The listing builds one solid part. Answer for the finished solid, in the listing's coordinates (mm). Face numbers are marked on the shaded views. Coordinates: 2 decimals unless noted, no trailing zeros. Loops run counter-clockwise (first coordinate to the right, second up) from the corner with the lowest first, then second, coordinate; pieces in that order, holes last. Notation, with made-up numbers: (81, 28.25) - (101, 28.25) arc R24 ccw to (101, 52.25) - close; hole circle Ø5 at (47.25, -9). An arc over 180 degrees is marked (long way). Return JSON: item names as keys, results as strings. Group by question number.
1. Each of these flat-tipped pins is pushed along its axis until it touches: P1, Ø1.3, axis at x = 9, y = -20, coming from the +Z side; P2, Ø11, axis at x = 2, y = 6.5, coming from the -Z side; P3, Ø1.9, axis at x = -10, y = -19, coming from the -Z side. Where does it stop, or does it pass through?
2. Section D-D (y = -2) is taken. Write down the section's boundary in (x, z).
3. The mould has two halves that part along X. Classify the marked faces 1 and 2: pulls with the +X half, pulls with the -X half, needs draft (parallel to the pull), parting line crosses it, or undercut.
4. Find the intervals of material crossed by line 1 along X through (y, z) = (-19, 2.45); line 2 along X through (y, z) = (-19, 7.45); line 3 along Y through (x, z) = (10, 6.6), in increasing order.
5. Section A-A (y = -19) is taken. Write down the section's boundary in (x, z) (3 decimals), and give its area (3 significant figures).
6. Section C-C (x = 0) is taken. Write down the section's boundary in (y, z), and give its area (3 significant figures).
7. Section B-B (z = 4) is taken. Write down the section's boundary in (x, y), and give its area (3 significant figures).
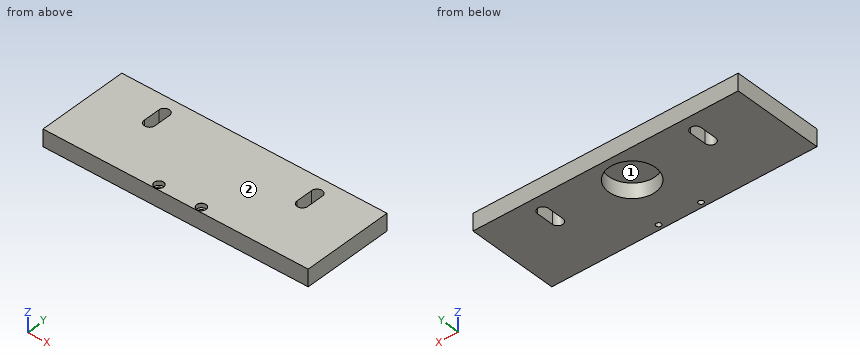
```python
from build123d import *

# Parameters (mm, degrees)
ESBO_O1_W                        = 125
ESBO_O1_H                        = 43
RESSALTO_EXTRUS_O1_DEPTH         = 8
CORTE_EXTRUS_O1_DEPTH            = 9
REBAIXO_PARA_SHCS_M21_AT_2_COUNT = 2
REBAIXO_PARA_SHCS_M21_AT_2_PITCH = 20
ESBO_O6_R                        = 11
CORTE_EXTRUS_O2_DEPTH            = 7


with BuildPart() as part:
    # Esboço1 → Ressalto-extrusão1 (new body)
    with BuildSketch(Plane.XY):
        Rectangle(ESBO_O1_W, ESBO_O1_H)
    extrude(amount=RESSALTO_EXTRUS_O1_DEPTH)

    # Esboço2 → Corte-extrusão1 (cut, through all)
    with BuildSketch(Plane.XY.offset(8)):
        with BuildLine():
            Line((-33.5, 6), (-33.5, 14))
            ThreePointArc((-33.5, 14), (-36, 16.5), (-38.5, 14))
            Line((-38.5, 14), (-38.5, 6))
            ThreePointArc((-38.5, 6), (-36, 3.5), (-33.5, 6))
        make_face()
        with BuildLine():
            Line((38.5, 6), (38.5, 14))
            ThreePointArc((38.5, 14), (36, 16.5), (33.5, 14))
            Line((33.5, 14), (33.5, 6))
            ThreePointArc((33.5, 6), (36, 3.5), (38.5, 6))
        make_face()
    extrude(amount=-CORTE_EXTRUS_O1_DEPTH, mode=Mode.SUBTRACT)

    # Esboço4 → Rebaixo para SHCS M21 (revolve, cut)
    with BuildSketch(Plane(origin=(-10, -19, 8), x_dir=(0, -1, 0), z_dir=(1, 0, 0))):
        Polygon((0, 0), (0, 8), (1.2, 8), (1.2, 2), (2.2, 2), (2.2, 0.025), (2.225, 0), align=None)
    rebaixo_para_shcs_m21 = revolve(axis=Axis((-10, -19, 14.35), (0, 0, -1)), mode=Mode.SUBTRACT)

    # Rebaixo para SHCS M21 at 2: Rebaixo para SHCS M21 ×2
    with Locations(*[(i * REBAIXO_PARA_SHCS_M21_AT_2_PITCH, 0, 0) for i in range(1, REBAIXO_PARA_SHCS_M21_AT_2_COUNT)]):
        add(rebaixo_para_shcs_m21, mode=Mode.SUBTRACT)

    # Esboço6 → Corte-extrusão2 (cut)
    with BuildSketch(Plane(origin=(0, 0, 0), x_dir=(-1, 0, 0), z_dir=(0, 0, -1))):
        with Locations((0, 7)):
            Circle(ESBO_O6_R)
    extrude(amount=-CORTE_EXTRUS_O2_DEPTH, mode=Mode.SUBTRACT)


solid = part.part
```
The answers:
{
 "1": {"P1": "stops at z = 6", "P2": "stops at z = 7", "P3": "passes through"},
 "2": {"outline": "(-62.5, 0) - (-6.32, 0) - (-6.32, 7) - (6.32, 7) - (6.32, 0) - (62.5, 0) - (62.5, 8) - (-62.5, 8) - close"},
 "3": {"face 1": "undercut", "face 2": "needs draft"},
 "4": {"line 1": "x = -62.5 to -11.2, -8.8 to 8.8, 11.2 to 62.5", "line 2": "x = -62.5 to -12.2, -7.8 to 7.8, 12.2 to 62.5", "line 3": "y = -21.5 to -21.2, -16.8 to 2.42, 11.58 to 21.5"},
 "5": {"outline": "(-62.5, 0) - (-11.2, 0) - (-11.2, 6) - (-12.2, 6) - (-12.2, 7.975) - (-12.225, 8) - (-62.5, 8) - close; (-8.8, 0) - (8.8, 0) - (8.8, 6) - (7.8, 6) - (7.8, 7.975) - (7.775, 8) - (-7.775, 8) - (-7.8, 7.975) - (-7.8, 6) - (-8.8, 6) - close; (11.2, 0) - (62.5, 0) - (62.5, 8) - (12.225, 8) - (12.2, 7.975) - (12.2, 6) - (11.2, 6) - close", "area": "954 mm2"},
 "6": {"outline": "(-21.5, 0) - (-4, 0) - (-4, 7) - (18, 7) - (18, 0) - (21.5, 0) - (21.5, 8) - (-21.5, 8) - close", "area": "190 mm2"},
 "7": {"outline": "(-62.5, -21.5) - (62.5, -21.5) - (62.5, 21.5) - (-62.5, 21.5) - close; hole (-38.5, 6) arc R2.5 ccw to (-33.5, 6) - (-33.5, 14) arc R2.5 ccw to (-38.5, 14) - close; hole circle Ø2.4 at (-10, -19); hole circle Ø22 at (0, 7); hole circle Ø2.4 at (10, -19); hole (33.5, 6) arc R2.5 ccw to (38.5, 6) - (38.5, 14) arc R2.5 ccw to (33.5, 14) - close", "area": "4,870 mm2"}
}
